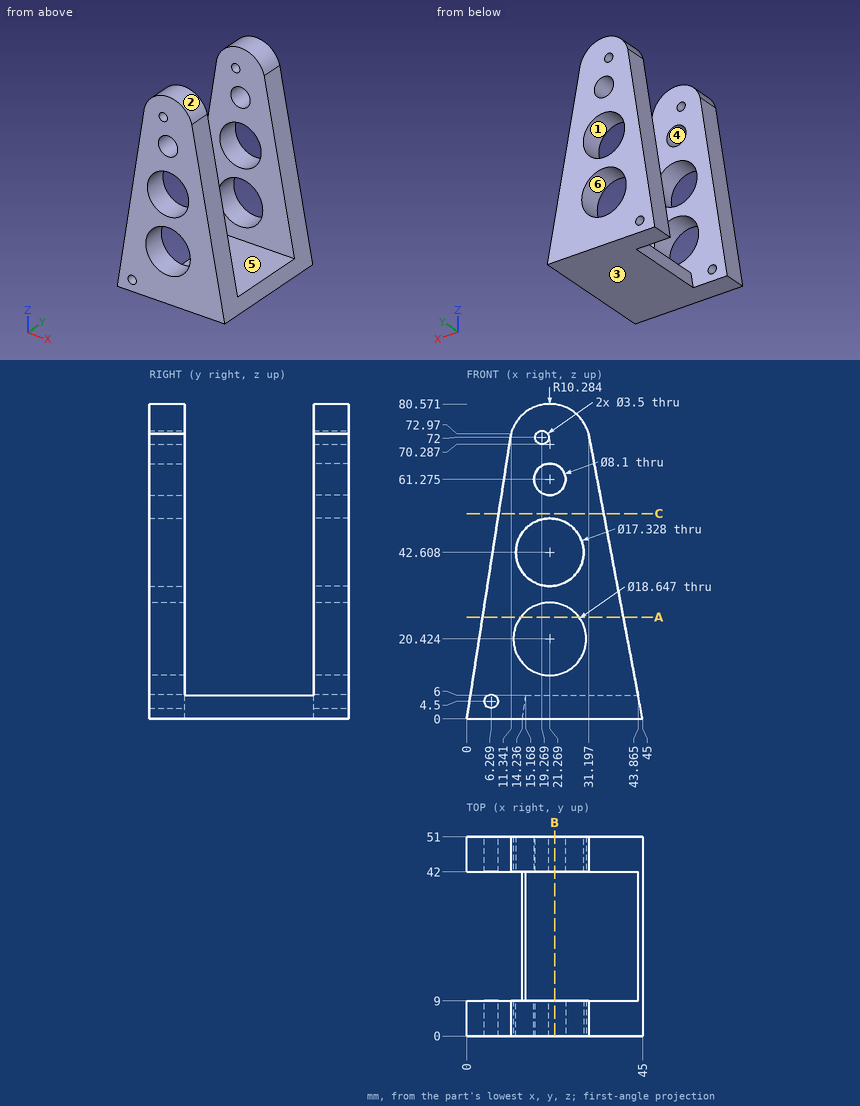
Geometry: see drawing. Coordinates: mm, zero at the bounding-box minimum. A direction names the side the tool comes from. Round coordinates to 2 decimals unless told otherwise and drop trailing zeros. Write each loop counter-clockwise with the first axis right and the second up, starting at its lowest first coordinate (ties: lowest second). Pieces come first, ordered by that corner, then holes. Notation, with made-up numbers: M 37.25,48 L 52.25,48 A22 cw 52.25,65 Z; hole C 21.25,77.5 d1. An arc over 180 degrees is marked long. Answer in a Markdown table with one row per item. Add a question column.
(1) Cut plane C-C, the plane z = 52.5. Return the cut outline in (x, y), then the cut area to 3 significant figures.
(2) Contact query for flat-ended pins moving along their axis: pin 1 (5 mm diameter, centred on x = 27.5, y = 13, fed in from +Z); pin 2 (8 mm diameter, centred on y = 12, z = 62, fed in from +X). Output: stop coordinate, or through.
(3) Reachability of the marked faces 5 and 6 from +Z, -Z, +X, -X, +Y, -Y: full face, straight path, thin tool, end or side. Return the list, or none.
(4) Ray query, L1, parallel to Y at x = 18, z = 69; L2, parallel to Z at x = 39, y = 18.5; L3, parallel to X at y = 46.5, z = 46. Return the intervals inside material, ascending.
(5) Draft query along X for the marked faces 1, 2, 3 and 4. Return one class per face: pulls with the +X half, pulls with the -X half, needs draft (parallel to the pull), parting line crosses it, or undercut.
(6) Cut plane A-A, the plane z = 26. Return the cut outline in (x, y).
(7) Cut plane B-B, the plane x = 22.5. Give the number of separate pieces and of enclosed holes in the cut face.
Established:
| question | item | result |
|---|---|---|
| 1 | outline | M 8.16,0 L 35.07,0 L 35.07,9 L 8.16,9 Z; M 8.16,42 L 35.07,42 L 35.07,51 L 8.16,51 Z |
| 1 | area | 484 mm² |
| 2 | pin 1 | z = 6 |
| 2 | pin 2 | x = 33.77 |
| 3 | face 5 | +Z, +X, -X |
| 3 | face 6 | +Y, -Y |
| 4 | L1 | 0 to 9, 42 to 51 |
| 4 | L2 | 0 to 6 |
| 4 | L3 | 7.15 to 13.3, 29.24 to 36.3 |
| 5 | face 1 | undercut |
| 5 | face 2 | parting line crosses it |
| 5 | face 3 | needs draft |
| 5 | face 4 | undercut |
| 6 | outline | M 4.04,0 L 13.8,0 L 13.8,9 L 4.04,9 Z; M 4.04,42 L 13.8,42 L 13.8,51 L 4.04,51 Z; M 28.74,0 L 40.08,0 L 40.08,9 L 28.74,9 Z; M 28.74,42 L 40.08,42 L 40.08,51 L 28.74,51 Z |
| 7 | separate pieces | 7 |
| 7 | enclosed holes | 0 |
